Design review of the part built by this model. Coordinates are the model's own, in mm. A direction names the side the tool comes from. Round coordinates to 2 decimals unless told otherwise and drop trailing zeros. Write each loop counter-clockwise with the first axis right and the second up, starting at its lowest first coordinate (ties: lowest second). Pieces come first, ordered by that corner, then holes. Notation, with made-up numbers: M 74.5,51.25 L 124.5,51.25 A14 ccw 124.5,61.25 Z; hole C 48.5,-1 d9. An arc over 180 degrees is marked long. One line per question, with ' | ' between items. Start each with the question number.
Item 1: Machinability: for faces 1 (the face through (-61, 16, 0)), 2 (the face through (-104, 22.468, 1)), 3 (the face through (7, 18.468, 1)), 4 (the face through (-112.475, 28, 1)), which of the approach directions +Z, -Z, +X, -X, +Y, -Y give a long, thin tool a straight path to every point of the face, cutting with its end or side? Answer none if there is none.
Item 2: Draft analysis for pull direction X (two halves, no side actions). For faces 5 (the face through (14.525, 27, 1)), 6 (the face through (6, 22.468, 1)), 7 (the face through (-48.88, 4.48, -3.94)), state which applies: released by +X, released by -X, zero draft, split by the parting line, or undercut.
Item 3: Add section C-C, the plane y = 14. State the section outline as (x, z) points, and give its area (3 significant figures).
Item 4: For L1, parallel to X at y = 23.5, z = 4; L2, parallel to Y at x = 3.5, z = 9.75; L3, parallel to Z at x = -48, y = 6.5, list the stretches that pass through material, from the lowest coordinate up.
Item 5: Insertion check: pin 1 Ø4 at (y, z) = (23, 2.5) entering from +X; pin 2 Ø18.5 at (x, y) = (-88.97, 18.47) entering from +Z; pin 3 Ø8 at (y, z) = (27.5, -2) entering from -X. Each pin has a flat end and moves straight along its axis. Give the tip position at first contact, or say it passes through.
Item 6: Add section D-D, the plane z = 7.75. State the section outline as (x, y) points.
Item 7: Add section B-B, the plane x = 4. State the section outline as (y, z) points, and give its area (3 significant figures).
Item 8: Add section A-A, the plane z = -3.5. State the section outline as (x, y) points.
```python
from build123d import *

# Parameters (mm, degrees)
F1_DEPTH = 8
F2_DEPTH = 10
F3_DEPTH = 10
F4_D     = 23
F5_DEPTH = 1
F6_DEPTH = 2


with BuildPart() as f1:
    # F0 (on Top) → F1 (new body)
    with BuildSketch(Plane.XY):
        with BuildLine():
            Line((-49.4748241749, 32.4677416086), (-114.4748240411, 32.4677416086))
            Line((-114.4748240411, 32.4677416086), (-114.4748240411, 22.4677416086))
            Line((-114.4748240411, 22.4677416086), (-95.9030272714, 22.4677416086))
            ThreePointArc((-95.9030272714, 22.4677416086), (-86.9042716803, 26.1951482189), (-80.9748240411, 18.4677416086))
            ThreePointArc((-80.9748240411, 18.4677416086), (-88.9748240411, 10.4677416086), (-96.9748240411, 18.4677416086))
            Line((-96.9748240411, 18.4677416086), (-114.4748240411, 18.4677416086))
            Line((-114.4748240411, 18.4677416086), (-114.4748240411, -3.5322583914))
            Line((-114.4748240411, -3.5322583914), (15.5251759589, -3.5322583914))
            Line((15.5251759589, -3.5322583914), (15.5251759589, 18.4677416086))
            Line((15.5251759589, 18.4677416086), (-1.9748240411, 18.4677416086))
            ThreePointArc((-1.9748240411, 18.4677416086), (-17.7022306514, 16.3971892478), (-3.0466208109, 22.4677416086))
            Line((-3.0466208109, 22.4677416086), (15.5251759589, 22.4677416086))
            Line((15.5251759589, 22.4677416086), (15.5251759589, 32.4677416086))
            Line((15.5251759589, 32.4677416086), (-49.4748241749, 32.4677416086))
        make_face()
        with BuildLine():
            ThreePointArc((-50.7033488202, 32.4137348277), (-50.0896797547, 32.4542333936), (-49.4748241749, 32.4677416086))
            ThreePointArc((-49.4748241749, 32.4677416086), (-48.8599684612, 32.4542333995), (-48.246299262, 32.4137348277))
            ThreePointArc((-48.246299262, 32.4137348277), (-39.1501122556, 27.9229161996), (-35.4748240411, 18.4677416086))
            ThreePointArc((-35.4748240411, 18.4677416086), (-58.9299986321, 8.1430298231), (-50.7033488202, 32.4137348277))
        make_face(mode=Mode.SUBTRACT)
        with BuildLine():
            ThreePointArc((-48.246299262, 32.4137348277), (-48.8599684612, 32.4542333995), (-49.4748241749, 32.4677416086))
            ThreePointArc((-49.4748241749, 32.4677416086), (-50.0896797547, 32.4542333936), (-50.7033488202, 32.4137348277))
            Line((-50.7033488202, 32.4137348277), (-48.246299262, 32.4137348277))
        make_face()
    extrude(amount=-F1_DEPTH)

    # F3 (add): a face of the model
    f3_faces = [f1.faces().sort_by_distance(p)[0] for p in [
        (6.7751759589, 17.1188161103, 0),
    ]]


with BuildPart() as f2:
    # F0 (on Top) → F2 (new body)
    with BuildSketch(Plane.XY):
        with BuildLine():
            ThreePointArc((-35.4748240411, 18.4677416086), (-39.1501122556, 27.9229161996), (-48.246299262, 32.4137348277))
            Line((-48.246299262, 32.4137348277), (-50.7033488202, 32.4137348277))
            ThreePointArc((-50.7033488202, 32.4137348277), (-58.9299986321, 8.1430298231), (-35.4748240411, 18.4677416086))
        make_face()
    extrude(amount=F2_DEPTH)


with BuildPart() as f1_1:
    add(f1.part)

    add(f2.part)  # F3 merges F2
    extrude(f3_faces, amount=F3_DEPTH)

    # F4 (through all)
    with Locations(Plane(origin=(0, 0, 0), x_dir=(1, 0, 0), z_dir=(0, 0, -1))):
        with Locations((-49.4748240411, -18.4677416086)):
            Hole(F4_D / 2)

    # F5 (cut, symmetric): faces of the model
    f5_faces = [f1_1.faces().sort_by_distance(p)[0] for p in [
        (15.5251759589, 27.4677416086, 1),
        (15.5251759589, 27.4677416086, 1),
    ]]
    extrude(f5_faces, amount=F5_DEPTH, both=True, mode=Mode.SUBTRACT)

    # F6 (cut): faces of the model
    f6_faces = [f1_1.faces().sort_by_distance(p)[0] for p in [
        (-114.4748240411, 27.4677416086, 1),
        (-114.4748240411, 27.4677416086, 1),
    ]]
    extrude(f6_faces, amount=-F6_DEPTH, mode=Mode.SUBTRACT)


solid = f1_1.part
```
Computed values:
1) face 1: -Z | face 2: +Z, -Z, -X | face 3: +Z, -Z, +X | face 4: +Z, -Z, -X, +Y
2) face 5: released by +X | face 6: zero draft | face 7: undercut
3) outline: M -114.47,-8 L -95.61,-8 L -95.61,10 L -114.47,10 Z; M -82.34,-8 L -62.74,-8 L -62.74,0 L -60.07,0 L -60.07,10 L -82.34,10 Z; M -38.88,0 L -36.21,0 L -36.21,-8 L -16.61,-8 L -16.61,10 L -38.88,10 Z; M -3.34,-8 L 15.53,-8 L 15.53,10 L -3.34,10 Z | area: 1,440 mm^2
4) L1: x = -112.47 to -95.19, -82.76 to -59.82, -39.13 to -16.19, -3.76 to 14.53 | L2: y = -3.53 to 18.47, 22.47 to 32.47 | L3: z = 0 to 10
5) pin 1: stops at x = 14.53 | pin 2: stops at z = 10 | pin 3: stops at x = -112.47
6) outline: M -114.47,-3.53 L 15.53,-3.53 L 15.53,18.47 L -1.97,18.47 A8 cw long -3.05,22.47 L 14.53,22.47 L 14.53,32.47 L -112.47,32.47 L -112.47,22.47 L -95.9,22.47 A8 cw long -96.97,18.47 L -114.47,18.47 Z; hole C -49.47,18.47 d23
7) outline: M -3.53,-8 L 18.47,-8 L 18.47,10 L -3.53,10 Z; M 22.47,-8 L 32.47,-8 L 32.47,10 L 22.47,10 Z | area: 576 mm^2
8) outline: M -114.47,-3.53 L 15.53,-3.53 L 15.53,18.47 L -1.97,18.47 A8 cw long -3.05,22.47 L 14.53,22.47 L 14.53,32.47 L -112.47,32.47 L -112.47,22.47 L -95.9,22.47 A8 cw long -96.97,18.47 L -114.47,18.47 Z; hole M -50.7,32.41 A14 ccw long -48.25,32.41 Z
